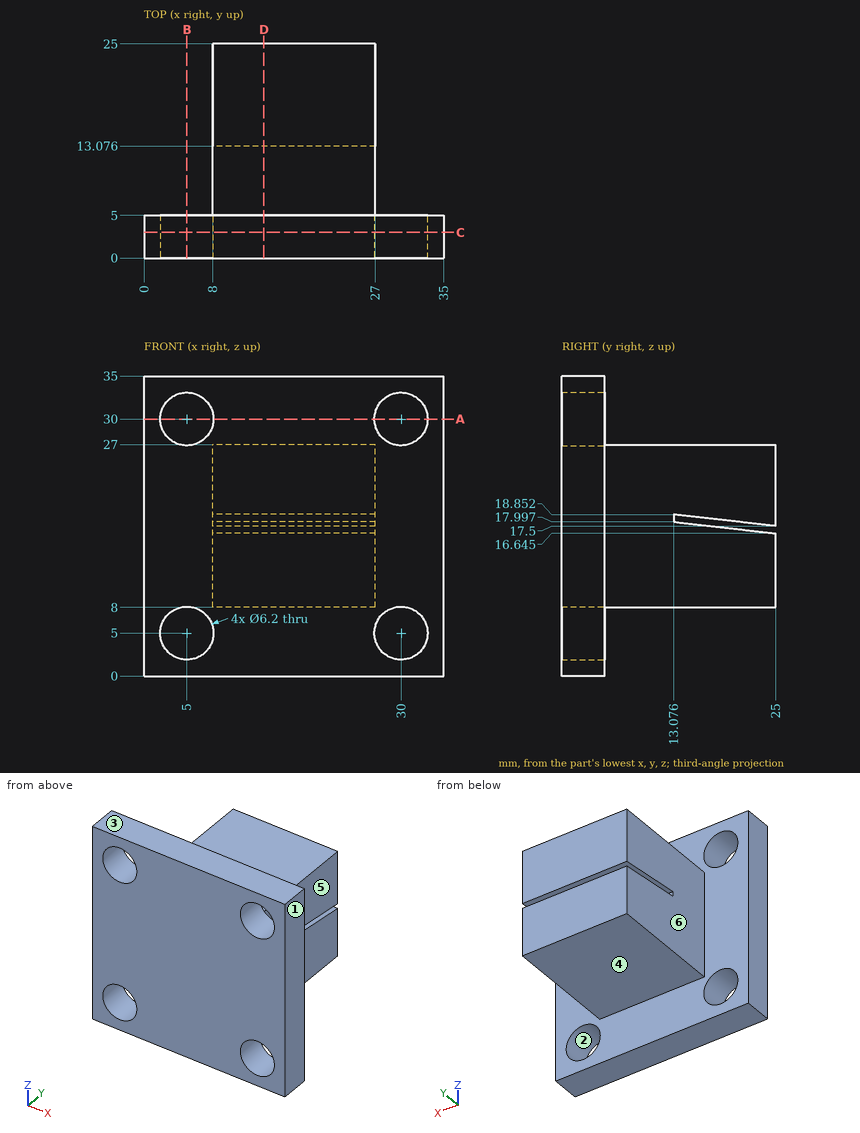
Verification items for this drawing (mm, ordinates from the low corner). A direction names the side the tool comes from. Give positions to 0.01 mm unless a question says otherwise; leave off trailing zeros. Write each loop counter-clockwise with the first axis right and the second up, starting at its lowest first coordinate (ties: lowest second). Pieces come first, ordered by that corner, then holes. Notation, with made-up numbers: (35, 82) -> (73, 82) arc R22 cw to (73, 102) -> close; hole circle Ø3 at (38.5, 86.25). An arc over 180 degrees is marked (long way). Use one line per item in the form item = value.
Item 1: Sectioned sample at C-C on y = 3. Enter the section's corners in (x, z), plus the area to 3 significant figures.
Results list:
outline = (0, 0) -> (35, 0) -> (35, 35) -> (0, 35) -> close; hole circle Ø6.2 at (5, 5); hole circle Ø6.2 at (5, 30); hole circle Ø6.2 at (30, 5); hole circle Ø6.2 at (30, 30)
area = 1,100 mm2
Item 2: Sectioned sample at D-D on x = 14. Enter the section's corners in (y, z) (1 decimal).
Results list:
outline = (0, 0) -> (5, 0) -> (5, 8) -> (25, 8) -> (25, 16.6) -> (13.1, 18) -> (13.1, 18.9) -> (25, 17.5) -> (25, 27) -> (5, 27) -> (5, 35) -> (0, 35) -> close
Item 3: Sectioned sample at A-A on z = 30. Enter the section's corners in (x, y), plus the area to 3 significant figures.
Results list:
outline = (0, 0) -> (1.9, 0) -> (1.9, 5) -> (0, 5) -> close; (8.1, 0) -> (26.9, 0) -> (26.9, 5) -> (8.1, 5) -> close; (33.1, 0) -> (35, 0) -> (35, 5) -> (33.1, 5) -> close
area = 113 mm2
Item 4: Mould release check, pull along X, two halves, no side actions. Record for the marked faces 1, 2 and 3: released by +X, released by -X, zero draft, split by the parting line, or undercut.
Results list:
face_1 = released by +X
face_2 = undercut
face_3 = zero draft
Item 5: Scan lines: line 1 (Z direction, x = 5, y = 1.4); line 2 (Z direction, x = 31, y = 1) (1 decimal); line 3 (Y direction, x = 23.5, z = 3). Record each from-to range of solid material in increasing order.
Results list:
line_1 = 0 to 1.9, 8.1 to 26.9, 33.1 to 35
line_2 = 0 to 2.1, 7.9 to 27.1, 32.9 to 35
line_3 = 0 to 5
Item 6: Sectioned sample at B-B on x = 5. Enter the section's corners in (y, z).
Results list:
outline = (0, 0) -> (5, 0) -> (5, 1.9) -> (0, 1.9) -> close; (0, 8.1) -> (5, 8.1) -> (5, 26.9) -> (0, 26.9) -> close; (0, 33.1) -> (5, 33.1) -> (5, 35) -> (0, 35) -> close
Item 7: Access from +Z, -Z, +X, -X, +Y, -Y to the whole of each face (thin tool, end or side, straight path). Record for the marked faces 4, 5 and 6.
Results list:
face_4 = -Z, +X, -X, +Y
face_5 = +Z, -Z, +X, +Y
face_6 = +Z, -Z, -X, +Y
Item 8: Depth check by flat-ended pin: pin 1 Ø8 at (x, y) = (25.5, 17) entering from -Z; pin 2 Ø8 at (x, z) = (5, 30) entering from +Y; pin 3 Ø5 at (y, z) = (15.5, 6.5) entering from -X. Enter the tip coordinate at first touch or a pass-through.
Results list:
pin_1 = 8
pin_2 = 5
pin_3 = 8
